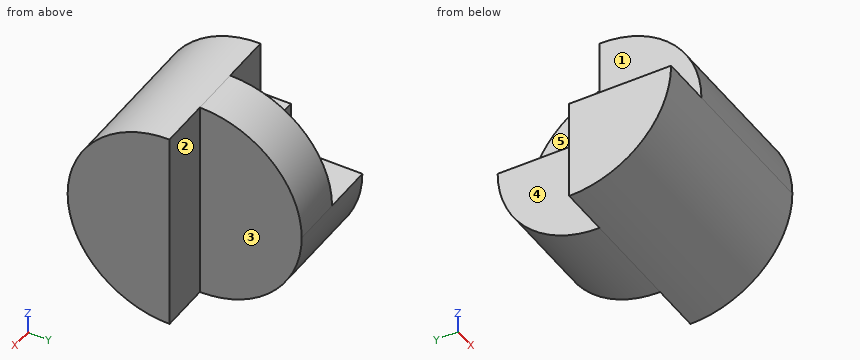
```python
from build123d import *

# Parameters (mm, degrees)
SKETCH1_W           = 40
SKETCH1_H           = 40
BOSS_EXTRUDE1_DEPTH = 40
SKETCH2_W           = 10
SKETCH2_H           = 20
CUT_EXTRUDE1_DEPTH  = 40
CUT_EXTRUDE2_DEPTH  = 40
CUT_EXTRUDE3_DEPTH  = 40
CUT_EXTRUDE4_DEPTH  = 10
CUT_EXTRUDE5_DEPTH  = 10


with BuildPart() as part:
    # Sketch1 → Boss-Extrude1 (new body)
    with BuildSketch(Plane.XY):
        with Locations((20, 20)):
            Rectangle(SKETCH1_W, SKETCH1_H)
    extrude(amount=BOSS_EXTRUDE1_DEPTH)

    # Sketch2 → Cut-Extrude1 (cut)
    with BuildSketch(Plane.XY.offset(40)):
        with Locations((5, 30)):
            Rectangle(SKETCH2_W, SKETCH2_H)
        with Locations((35, 30)):
            Rectangle(SKETCH2_W, SKETCH2_H)
    extrude(amount=-CUT_EXTRUDE1_DEPTH, mode=Mode.SUBTRACT)

    # Sketch3 → Cut-Extrude2 (cut)
    with BuildSketch(Plane.ZY):
        with BuildLine():
            ThreePointArc((20, 0), (5.857864376, 5.857864376), (0, 20))
            Line((0, 20), (0, 0))
            Line((0, 0), (20, 0))
        make_face()
        with BuildLine():
            ThreePointArc((40, 20), (34.142135624, 5.857864376), (20, 0))
            Line((20, 0), (40, 0))
            Line((40, 0), (40, 20))
        make_face()
    extrude(amount=-CUT_EXTRUDE2_DEPTH, mode=Mode.SUBTRACT)

    # Sketch4 → Cut-Extrude3 (cut)
    with BuildSketch(Plane.ZY.offset(-10)):
        with BuildLine():
            Line((0, 40), (0, 20))
            ThreePointArc((0, 20), (5.857864376, 34.142135624), (20, 40))
            Line((20, 40), (0, 40))
        make_face()
        with BuildLine():
            Line((40, 40), (20, 40))
            ThreePointArc((20, 40), (34.142135624, 34.142135624), (40, 20))
            Line((40, 20), (40, 40))
        make_face()
    extrude(amount=-CUT_EXTRUDE3_DEPTH, mode=Mode.SUBTRACT)

    # Sketch5 → Cut-Extrude4 (cut)
    with BuildSketch(Plane.ZY):
        with BuildLine():
            Line((20, 0), (20, 20))
            Line((20, 20), (40, 20))
            ThreePointArc((40, 20), (34.142135624, 5.857864376), (20, 0))
        make_face()
    extrude(amount=-CUT_EXTRUDE4_DEPTH, mode=Mode.SUBTRACT)

    # Sketch6 → Cut-Extrude5 (cut)
    with BuildSketch(Plane.ZY.offset(-10)):
        with BuildLine():
            Line((20, 40), (20, 20))
            Line((20, 20), (40, 20))
            ThreePointArc((40, 20), (34.142135624, 34.142135624), (20, 40))
        make_face()
    extrude(amount=-CUT_EXTRUDE5_DEPTH, mode=Mode.SUBTRACT)


solid = part.part
```
The model under review builds one solid part; all positions refer to its coordinate system, in mm. Face numbers are marked on the shaded views. A direction names the side the tool comes from. Round coordinates to 2 decimals unless told otherwise and drop trailing zeros. Order: outer loops, then holes, each group sorted by start corner. A loop starts at its lowest first (then second) coordinate and runs counter-clockwise, first axis right, second up. Notation, with made-up numbers: (54, 55.5) - (68, 55.5) arc R18 ccw to (68, 67.5) - close; hole circle Ø7 at (-31.75, 68). An arc over 180 degrees is marked (long way). Answer in a Markdown table with one row per item.
(1) Mouldability with a two-part tool opening along Y and no side actions: class the marked faces 1 and 2 as released by +Y, released by -Y, zero draft, split by the parting line, or undercut.
Result set:
| item | result |
|---|---|
| face 1 | zero draft |
| face 2 | released by +Y |
(2) Machinability: for the marked faces 3, 4 and 5, which of the approach directions +Z, -Z, +X, -X, +Y, -Y give a long, thin tool a straight path to every point of the face, cutting with its end or side? Answer none if there is none.
Result set:
| item | result |
|---|---|
| face 3 | +Z, -Z, +X, +Y |
| face 4 | +Z, -Z, -X, +Y |
| face 5 | +Z, -X, +Y |
(3) For line 1 (X direction, y = 8, z = 24.5); line 2 (X direction, y = 25, z = 2); line 3 (Y direction, x = 7.5, z = 19.5), list the stretches that pass through material, from the lowest coordinate up. Write a range as from..to.
Result set:
| item | result |
|---|---|
| line 1 | x = 10..40 |
| line 2 | x = 10..30 |
| line 3 | y = 0.01..20 |
(4) Take a section at C-C on y = 11. Write out the cut boundary in (x, z).
Result set:
| item | result |
|---|---|
| outline | (0, 2.14) - (40, 2.14) - (40, 37.86) - (10, 37.86) - (10, 20) - (0, 20) - close |
(5) Take a section at D-D on z = 36. Write out the cut boundary in (x, y), plus the area to 3 significant figures.
Result set:
| item | result |
|---|---|
| outline | (10, 8) - (40, 8) - (40, 20) - (30, 20) - (30, 32) - (20, 32) - (20, 20) - (10, 20) - close |
| area | 480 mm2 |
(6) Clearance check with flat-ended pins moving along their axes: P1, Ø3, axis at x = 4, y = 6.5, coming from the +Z side; P2, Ø22, axis at y = 34, z = 9.5, coming from the -X side; P3, Ø8, axis at x = 3, z = 5.5, coming from the +Y side. State where each tip first meets the part, or that it passes through.
Result set:
| item | result |
|---|---|
| P1 | stops at z = 20 |
| P2 | stops at x = 10 |
| P3 | stops at y = 20 |
(7) Take a section at A-A on z = 25.5. Write out the cut boundary in (x, y).
Result set:
| item | result |
|---|---|
| outline | (10, 0.77) - (40, 0.77) - (40, 20) - (30, 20) - (30, 39.23) - (20, 39.23) - (20, 20) - (10, 20) - close |
(8) Take a section at B-B on x = 11. Write out the cut boundary in (y, z).
Result set:
| item | result |
|---|---|
| outline | (20, 20) - (20, 40) arc R20 ccw (long way) to (40, 20) - close |
